```python
from build123d import *

# Parameters (mm, degrees)
SKETCH_1_W          = 10
SKETCH_1_H          = 10
SKETCH_1_W_2        = 8
SKETCH_1_H_2        = 8
EXTRUDE_1_DEPTH     = 39.4
SKETCH_2_R          = 1.6
CUT_EXTRUDE_1_DEPTH = 41.9555857
SKETCH_3_R          = 1.6
CUT_EXTRUDE_2_DEPTH = 41.9555857
SKETCH_4_R          = 1.6
CUT_EXTRUDE_3_DEPTH = 41.9555857


with BuildPart() as part:
    # ｽｹｯﾁ1 → 押し出し-薄板1 (new body)
    with BuildSketch(Plane.XY):
        Rectangle(SKETCH_1_W, SKETCH_1_H)
        Rectangle(SKETCH_1_W_2, SKETCH_1_H_2, mode=Mode.SUBTRACT)
    extrude(amount=EXTRUDE_1_DEPTH)

    # ｽｹｯﾁ2 → ｶｯﾄ - 押し出し1 (cut, through all)
    with BuildSketch(Plane(origin=(0, 5, 0), x_dir=(1, 0, 0), z_dir=(0, 1, 0))):
        with Locations(Location((0, -5, 0), (0, 0, 270))):
            Circle(SKETCH_2_R)
        with Locations(Location((0, -34.4, 0), (0, 0, 270))):
            Circle(SKETCH_2_R)
    extrude(amount=-CUT_EXTRUDE_1_DEPTH, mode=Mode.SUBTRACT)

    # ｽｹｯﾁ3 → ｶｯﾄ - 押し出し2 (cut, through all)
    with BuildSketch(Plane(origin=(0, 5, 0), x_dir=(1, 0, 0), z_dir=(0, 1, 0))):
        with Locations(Location((0, -13.75, 0), (0, 0, 270))):
            Circle(SKETCH_3_R)
        with Locations(Location((0, -25.65, 0), (0, 0, 270))):
            Circle(SKETCH_3_R)
    extrude(amount=-CUT_EXTRUDE_2_DEPTH, mode=Mode.SUBTRACT)

    # ｽｹｯﾁ4 → ｶｯﾄ - 押し出し3 (cut, through all)
    with BuildSketch(Plane(origin=(5, 0, 0), x_dir=(0, 0, -1), z_dir=(1, 0, 0))):
        with Locations((-19.7, 0)):
            Circle(SKETCH_4_R)
    extrude(amount=-CUT_EXTRUDE_3_DEPTH, mode=Mode.SUBTRACT)


solid = part.part
```
Part model, mm, in its own coordinate system. A direction names the side the tool comes from. Give positions to 0.01 mm unless a question says otherwise; leave off trailing zeros. Write each loop counter-clockwise with the first axis right and the second up, starting at its lowest first coordinate (ties: lowest second). Pieces come first, ordered by that corner, then holes. Notation, with made-up numbers: (40.25, 2) -> (74.25, 2) arc R13 ccw to (74.25, 24) -> close; hole circle Ø11 at (39, 34). An arc over 180 degrees is marked (long way). Put each result on its own line as item: value. Start each with the question number.
Item 1: Cut at A-A (y = 0). List the corners of the cut face in (x, z).
Item 2: Which spindle directions (+Z, -Z, +X, -X, +Y, -Y) get a long thin tool onto all of the face, cutting with end or side? Do faces 4 (the face through (0, 4, 19)), 5 (the face through (0.07, -4.49, 12.15)). Say none if no direction does.
Item 3: Pull direction Y, two halves, no side cores. Call faces 1 (the face through (0, -4, 19)), 2 (the face through (0.07, 4.51, 12.15)), 3 (the face through (0, 5, 19)): pulls with the +Y half, pulls with the -Y half, needs draft (parallel to the pull), parting line crosses it, or undercut.
Item 4: Wall check: L1, parallel to Y at x = 3.5, z = 20.5; L2, parallel to X at y = 4.7, z = 34.4. Give the ranges that are in metal, low to high. Write a range as [from, to].
Item 5: Pin check, flat tips, straight feed: pin 1 Ø4 at (x, z) = (0, 5) entering from +Y; pin 2 Ø2.5 at (y, z) = (0, 19.7) entering from -X. Stop position of each tip, or through.
Item 6: Cut at B-B (z = 10). List the corners of the cut face in (x, y).
Item 7: Cut at D-D (y = 2.5). List the corners of the cut face in (x, z), then the cut area to 3 significant figures.
Item 8: Cut at C-C (z = 25.65). List the corners of the cut face in (x, y), then the cut area to 3 significant figures.
Answer list:
1. outline: (-5, 0) -> (-4, 0) -> (-4, 18.1) -> (-5, 18.1) -> close; (-5, 21.3) -> (-4, 21.3) -> (-4, 39.4) -> (-5, 39.4) -> close; (4, 0) -> (5, 0) -> (5, 18.1) -> (4, 18.1) -> close; (4, 21.3) -> (5, 21.3) -> (5, 39.4) -> (4, 39.4) -> close
2. face 4: +Z, -Z
2. face 5: +Y, -Y
3. face 1: undercut
3. face 2: needs draft
3. face 3: pulls with the +Y half
4. L1: y = [-5, -4], [4, 5]
4. L2: x = [-5, -1.6], [1.6, 5]
5. pin 1: stops at y = 5
5. pin 2: passes through
6. outline: (-5, -5) -> (5, -5) -> (5, 5) -> (-5, 5) -> close; hole (-4, -4) -> (4, -4) -> (4, 4) -> (-4, 4) -> close
7. outline: (-5, 0) -> (-4, 0) -> (-4, 39.4) -> (-5, 39.4) -> close; (4, 0) -> (5, 0) -> (5, 39.4) -> (4, 39.4) -> close
7. area: 78.8 mm2
8. outline: (-5, -5) -> (-1.6, -5) -> (-1.6, -4) -> (-4, -4) -> (-4, 4) -> (-1.6, 4) -> (-1.6, 5) -> (-5, 5) -> close; (1.6, -5) -> (5, -5) -> (5, 5) -> (1.6, 5) -> (1.6, 4) -> (4, 4) -> (4, -4) -> (1.6, -4) -> close
8. area: 29.6 mm2
